Can you work these out from the model? Positions are in its coordinate system, mm. Round coordinates to 2 decimals unless told otherwise and drop trailing zeros. Write each loop counter-clockwise with the first axis right and the second up, starting at its lowest first coordinate (ties: lowest second). Pieces come first, ordered by that corner, then holes. Notation, with made-up numbers: M 89.25,38 L 100.25,38 A28 cw 100.25,59 Z; hole C -40,-38.75 d4. An arc over 180 degrees is marked long. Use one line per item in the form item = value. Start each with the question number.
```python
from build123d import *

# Parameters (mm, degrees)
CYLINDER024_R          = 5
CYLINDER024_DEPTH      = 5
CYLINDER024_ROLL_ANGLE = 90
BOX031_W               = 8
BOX031_H               = 5
BOX031_DEPTH           = 16
CYLINDER023_R          = 8
CYLINDER023_DEPTH      = 5
CYLINDER023_ROLL_ANGLE = 90


with BuildPart() as zylinder010:
    # Cylinder024 → Cylinder024 (new body)
    with BuildSketch(Plane.XY):
        Circle(CYLINDER024_R)
    extrude(amount=CYLINDER024_DEPTH)


with BuildPart() as zylinder010_1:
    # Cylinder024 roll: moved
    add(zylinder010.part.rotate(Axis((0, 0, 0), (1, 0, 0)), CYLINDER024_ROLL_ANGLE))


with BuildPart() as zylinder010_2:
    # Cylinder024 placement: moved
    add(zylinder010_1.part.moved(Location((8, 5, 8))))


with BuildPart() as obj1:
    # Box031 → Box031 (new body)
    with BuildSketch(Plane.XY):
        with Locations((4, 2.5)):
            Rectangle(BOX031_W, BOX031_H)
    extrude(amount=BOX031_DEPTH)


with BuildPart() as obj2:
    # Cylinder023 → Cylinder023 (new body)
    with BuildSketch(Plane.XY):
        Circle(CYLINDER023_R)
    extrude(amount=CYLINDER023_DEPTH)


with BuildPart() as obj2_1:
    # Cylinder023 roll: moved
    add(obj2.part.rotate(Axis((0, 0, 0), (1, 0, 0)), CYLINDER023_ROLL_ANGLE))


with BuildPart() as obj2_2:
    # Cylinder023 placement: moved
    add(obj2_1.part.moved(Location((8, 5, 8))))

    # Fusion016: union obj1
    add(obj1.part)

    # Cut021: cut Zylinder010
    add(zylinder010_2.part, mode=Mode.SUBTRACT)


with BuildPart() as obj2_3:
    # Cut021 placement: moved
    add(obj2_2.part.moved(Location((160, 70, 20))))


solid = obj2_3.part
```
1. Please list where these lines run through material, in increasing order: line 1 along Z through (x, y) = (168, 74); line 2 along X through (y, z) = (71.2, 29.75); line 3 along X through (y, z) = (70.4, 31).
2. If we section it at D-D (z = 34.5): List the corners of the cut face in (x, y) for me.
3. If we section it at A-A (z = 28): List the corners of the cut face in (x, y) for me, and give its area (3 significant figures).
4. If we section it at C-C (y = 72.2): List the corners of the cut face in (x, z) for me, and give its area (3 significant figures).
5. If we section it at B-B (x = 167): List the corners of the cut face in (y, z) for me, and give its area (3 significant figures).
6. Will these pins go through, and if not, where does the flat tip stop? pin 1 (1.5 mm diameter, centred on x = 173.5, y = 73.5, fed in from -Z); pin 2 (1.5 mm diameter, centred on y = 71.5, z = 26.5, fed in from +X).
7. If we mould it in two halves opening along Z, with no side actions, what happens to faces 1 (the face through (162.6, 70, 27.9)), 2 (the face through (176, 73, 28)), 3 (the face through (164, 73, 25))? For each: pulls with the +Z half, pulls with the -Z half, needs draft (parallel to the pull), parting line crosses it, or undercut.
Model answer:
q1.line_1 = 20 to 23, 33 to 36
q1.line_2 = 160 to 163.32, 172.68 to 175.81
q1.line_3 = 160 to 164, 172 to 175.42
q2.outline = M 160,70 L 172.66,70 L 172.66,75 L 160,75 Z
q3.outline = M 160,70 L 163,70 L 163,75 L 160,75 Z; M 173,70 L 176,70 L 176,75 L 173,75 Z
q3.area = 30.0 mm2
q4.outline = M 160,20 L 168,20 A8 ccw 168,36 L 160,36 Z; hole C 168,28 d10
q4.area = 150 mm2
q5.outline = M 70,20 L 75,20 L 75,23.1 L 70,23.1 Z; M 70,32.9 L 75,32.9 L 75,36 L 70,36 Z
q5.area = 31.0 mm2
q6.pin_1 = 21.56
q6.pin_2 = 175.96
q7.face_1 = needs draft
q7.face_2 = parting line crosses it
q7.face_3 = undercut
